Geometry: final body of the model. Coordinates: model frame, mm. Give positions to 0.01 mm unless a question says otherwise; leave off trailing zeros. Loops run counter-clockwise (first coordinate to the right, second up) from the corner with the lowest first, then second, coordinate; pieces in that order, holes last.
1. First-contact query: P1, Ø5, axis at y = 95, z = 443, coming from the +X side; P2, Ø4, axis at x = 1000.5, z = 395, coming from the -Y side; P3, Ø12, axis at y = 7.5, z = 262, coming from the +X side. Flat tips, straight axial feed; report the tip coordinate or a pass-through.
2. Section A-A, the plane z = 64. Output: boundary loops of the cut face in (x, y), then the cut area to 3 significant figures.
3. Section B-B, the plane z = 228.5. Output: boundary loops of the cut face in (x, y).
4. Material intervals for line 1 along Y through (x, z) = (46.5, 317); line 2 along X through (y, z) = (1304.5, 303.5); line 3 along X through (y, z) = (-199, 200.5), sorted ascending.
from build123d import *

# Parameters (mm, degrees)
F1_DEPTH = 550
F2_R     = 2500
F3_R     = 400


with BuildPart() as f1:
    # F0 (on Top) → F1 (new body)
    with BuildSketch(Plane.XY):
        with BuildLine():
            Line((0, 1620), (0, 698.7895697045))
            ThreePointArc((0, 698.7895697044), (402.0654375, 806.203125), (804.130875, 698.7895697044))
            Line((804.130875, 698.7895697044), (804.130875, 1620))
            Line((804.130875, 1620), (0, 1620))
        make_face()
        with BuildLine():
            Line((0, 698.7895697045), (0, 0))
            Line((0, 0), (804.130875, 0))
            Line((804.130875, 0), (804.130875, 698.7895697044))
            ThreePointArc((804.130875, 698.7895697044), (402.0654375, 806.203125), (0, 698.7895697044))
        make_face()
        with BuildLine():
            Line((804.130875, 0), (0, 0))
            Line((0, 0), (0, 698.7895697045))
            ThreePointArc((0, 698.7895697044), (-1.5538550225, -697.8932192416), (1208.2685625, 0))
            ThreePointArc((1208.2685625, 0), (1099.9586567416, 403.6192925225), (804.130875, 698.7895697044))
            Line((804.130875, 698.7895697044), (804.130875, 0))
        make_face()
    extrude(amount=F1_DEPTH)

    # F2
    f2_edges = [f1.edges().sort_by_distance(p)[0] for p in [
        (0, 698.78957, 275),
        (804.130875, 698.78957, 275),
    ]]
    fillet(f2_edges, radius=F2_R)

    # F3
    f3_edges = [f1.edges().sort_by_distance(p)[0] for p in [
        (881.732912, 965.928975, 550),
        (402.065437, -806.203125, 550),
        (-77.602037, 965.928975, 550),
    ]]
    fillet(f3_edges, radius=F3_R)


solid = f1.part
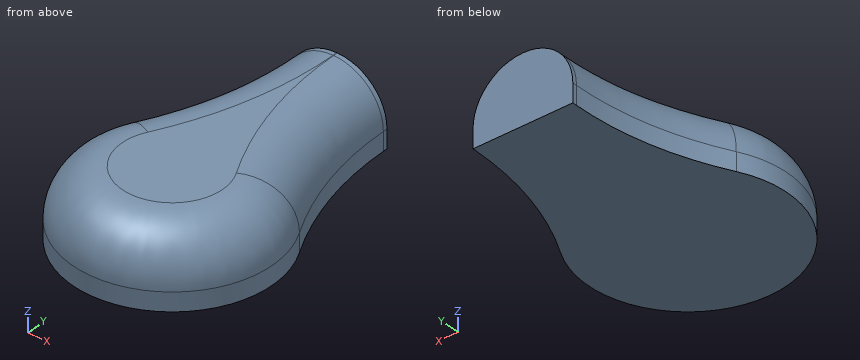
Answers below:
1. P1: stops at x = 1076.6
1. P2: stops at y = -408.65
1. P3: stops at x = 1193.93
2. outline: (-305.59, 386.25) arc R806.2 ccw (long way) to (1109.72, 386.25) arc R2500 cw to (804.13, 1583.98) - (804.13, 1620) - (0, 1620) - (0, 1583.98) arc R2500 cw to start
2. area: 2,850,000 mm2
3. outline: (-298.76, 382.52) arc R798.42 ccw (long way) to (1102.89, 382.52) arc R2507.78 cw to (796.35, 1583.98) - (796.35, 1620) - (7.78, 1620) - (7.78, 1583.98) arc R2507.78 cw to start
4. line 1: y = -682.62 to 1620
4. line 2: x = 15.14 to 788.99
4. line 3: x = -375.89 to 1180.02
